For this review, take the finished solid that the model builds, in its own axes (mm). A direction names the side the tool comes from. Give positions to 0.01 mm unless a question says otherwise; leave off trailing zeros. Loops run counter-clockwise (first coordinate to the right, second up) from the corner with the lowest first, then second, coordinate; pieces in that order, holes last. Notation, with made-up numbers: (65, 28) - (84, 28) arc R9 ccw to (84, 35) - close; hole circle Ø7 at (-39.75, 22.25). An arc over 180 degrees is marked (long way). Put each result on its own line as item: value.
Autodesk Inventor part; units mm, degrees
ref_plane "YZ Plane" through (0, 0, 0) normal (1, 0, 0) x (0, 1, 0)
ref_plane "XZ Plane" through (0, 0, 0) normal (0, 1, 0) x (-1, 0, 0)
ref_plane "XY Plane" through (0, 0, 0) normal (0, 0, 1) x (1, 0, 0)
sketch "Sketch1" plane through (0, 0, 0) normal (1, 0, 0) x (0, 1, 0)
  circle A0 centre (6.2867, -6.541) radius 3
  line L0 (6.2867, -9.541) -> (1, -9.541)
  line L1 (0, -8.541) -> (0, 0.5151)
  line L2 (0.785, 0.926) -> (7.9965, -4.0759)
  arc A1 (0.785, 0.926) -> (0, 0.5151) centre (0.5, 0.5151) ccw
  arc A2 (0, -8.541) -> (1, -9.541) centre (1, -8.541) ccw
  point P0 (0, 0)
  dimension "d0" = 6
  dimension "d1" = 0.5
  dimension "d2" = 1
extrude "Extrusion1" add sketch "Sketch1" along normal blind 10
shell "Shell1" thickness 0.5 removed faces 0
sketch "Sketch2" plane through (0, 0.785, 0.926) normal (0, 0.5699242, 0.8216972) x (1, 0, 0)
  line L0 (0, 8.7764) -> (0, 0)
  line L1 (0, 0) -> (10, 0)
  line L2 (10, 8.7764) -> (10, 0)
  line L3 (0, 8.7764) -> (10, 8.7764)
  line L4 (1.2, 7.3764) -> (8.8, 7.3764)
  line L5 (8.8, 7.3764) -> (8.8, 4.4678)
  line L6 (8.8, 4.4678) -> (1.2, 4.4678)
  line L7 (1.2, 4.4678) -> (1.2, 7.3764)
  circle A0 centre (1.94, 3.259) radius 0.5615
  circle A1 centre (1.94, 1.3767) radius 0.3
  circle A2 centre (2.8563, 1.3767) radius 0.3
  point P0 (0, -0.1173)
  dimension "d6" = 1.4
  dimension "d7" = 1.2
  dimension "d8" = 1.2
  dimension "d9" = 0.6
  dimension "d10" = 0.6
extrude "Extrusion2" cut sketch "Sketch2" against normal blind 0.2 contours L4 L5 L6 L7 | A0 | A1 | A2
sketch "Sketch3" plane through (0, 1, -9.541) normal (0, 0, -1) x (-1, 0, 0)
  circle A0 centre (-5, 2.6434) radius 0.7
  line L0 (0, 0) -> (0, 5.2867)
  line L1 (0, 5.2867) -> (-10, 5.2867)
  line L2 (-10, 0) -> (-10, 5.2867)
  line L3 (0, 0) -> (-10, 0)
  point P0 (0, -1)
  dimension "d13" = 1.4
extrude "Extrusion3" cut sketch "Sketch3" against normal blind 1 contours A0
properties part number "caja del arduino"
1) Take a section at C-C on y = 8.5. State the section outline as (x, z) points.
Geometry check:
outline: (0, -8.57) - (10, -8.57) - (10, -4.52) - (0, -4.52) - close; hole (0.5, -7.7) - (9.5, -7.7) - (9.5, -5.38) - (0.5, -5.38) - close
2) Wall thickness on line 1 (X direction, y = 6, z = -7.75); line 2 (Z direction, x = 7, y = 3.5); line 3 (Z direction, x = 6, y = 4.5): over which ranges is each line inside the solid? List them lowest first.
Geometry check:
line 1: x = 0 to 0.5, 9.5 to 10
line 2: z = -9.54 to -9.04, -1.57 to -0.96
line 3: z = -9.54 to -9.04, -2.26 to -1.9
3) Take a section at B-B on z = -5.5. State the section outline as (x, y) points.
Geometry check:
outline: (0, 0) - (10, 0) - (10, 9.1) - (0, 9.1) - close; hole (0.5, 0.5) - (9.5, 0.5) - (9.5, 8.56) - (0.5, 8.56) - close
4) Draft analysis for pull direction Z (two halves, no side actions). For faces 4 (the face through (4.93, 9.165, -7.386)), 5 (the face through (4.93, 3.539, -0.984)), 6 (the face through (6, 4, -9.041)), state which applies: pulls with the +Z half, pulls with the -Z half, needs draft (parallel to the pull), parting line crosses it, or undercut.
Geometry check:
face 4: parting line crosses it
face 5: pulls with the +Z half
face 6: undercut
5) For faces 1 (the face through (4, 4, -9.541)), 2 (the face through (5.516, 4.116, -9.295)), 3 (the face through (4.9, 8.7, -7.2)), list the 3-axis set-ups (+Z, -Z, +X, -X, +Y, -Y) from which the entire face can be reached by the end or side of a thin tool; tool diameter is ignored.
Geometry check:
face 1: -Z, +X, -X, +Y, -Y
face 2: -Z
face 3: none
